For this review, take the finished solid that the model builds, in its own axes (mm). A direction names the side the tool comes from. Round coordinates to 2 decimals unless told otherwise and drop trailing zeros. Write each loop counter-clockwise with the first axis right and the second up, starting at its lowest first coordinate (ties: lowest second). Pieces come first, ordered by that corner, then holes.
from build123d import *

# Parameters (mm, degrees)
SKETCH1_R           = 40
SKETCH1_R_2         = 5
BOSS_EXTRUDE1_DEPTH = 5
SKETCH2_R           = 40
SKETCH2_R_2         = 38.5
SKETCH2_R_3         = 3
BOSS_EXTRUDE2_DEPTH = 15
SKETCH5_R           = 4
CUT_EXTRUDE1_DEPTH  = 5


with BuildPart() as part:
    # Sketch1 → Boss-Extrude1 (new body)
    with BuildSketch(Plane(origin=(0, 0, 0), x_dir=(1, 0, 0), z_dir=(0, 1, 0))):
        with Locations(Location((0, 0, 0), (0, 0, 270))):
            Circle(SKETCH1_R)
        with Locations(Location((-21, 21, 0), (0, 0, 270))):
            Circle(SKETCH1_R_2, mode=Mode.SUBTRACT)
        with Locations(Location((-21, -21, 0), (0, 0, 270))):
            Circle(SKETCH1_R_2, mode=Mode.SUBTRACT)
        with Locations(Location((21, -21, 0), (0, 0, 270))):
            Circle(SKETCH1_R_2, mode=Mode.SUBTRACT)
        with Locations(Location((21, 21, 0), (0, 0, 270))):
            Circle(SKETCH1_R_2, mode=Mode.SUBTRACT)
    extrude(amount=BOSS_EXTRUDE1_DEPTH)

    # Sketch2 → Boss-Extrude2 (add)
    # profile 1 of 7: a face of its own
    with BuildSketch(Plane(origin=(0, 5, 0), x_dir=(1, 0, 0), z_dir=(0, 1, 0))):
        with Locations(Location((0, 0, 0), (0, 0, 270))):
            Circle(SKETCH2_R)
        with Locations(Location((0, 0, 0), (0, 0, 270))):
            Circle(SKETCH2_R_2, mode=Mode.SUBTRACT)
    # profile 2 of 7: a face of its own
    with BuildSketch(Plane(origin=(0, 5, 0), x_dir=(1, 0, 0), z_dir=(0, 1, 0))):
        with Locations(Location((-12, -21, 0), (0, 0, 270))):
            Circle(SKETCH2_R_3)
    # profile 3 of 7: a face of its own
    with BuildSketch(Plane(origin=(0, 5, 0), x_dir=(1, 0, 0), z_dir=(0, 1, 0))):
        with Locations(Location((12, -21, 0), (0, 0, 270))):
            Circle(SKETCH2_R_3)
    # profile 4 of 7: a face of its own
    with BuildSketch(Plane(origin=(0, 5, 0), x_dir=(1, 0, 0), z_dir=(0, 1, 0))):
        with Locations(Location((21, -12, 0), (0, 0, 270))):
            Circle(SKETCH2_R_3)
    # profile 5 of 7: a face of its own
    with BuildSketch(Plane(origin=(0, 5, 0), x_dir=(1, 0, 0), z_dir=(0, 1, 0))):
        with Locations(Location((21, 12, 0), (0, 0, 270))):
            Circle(SKETCH2_R_3)
    # profile 6 of 7: a face of its own
    with BuildSketch(Plane(origin=(0, 5, 0), x_dir=(1, 0, 0), z_dir=(0, 1, 0))):
        with Locations(Location((12, 21, 0), (0, 0, 270))):
            Circle(SKETCH2_R_3)
    # profile 7 of 7: a face of its own
    with BuildSketch(Plane(origin=(0, 5, 0), x_dir=(1, 0, 0), z_dir=(0, 1, 0))):
        with Locations(Location((-12, 21, 0), (0, 0, 270))):
            Circle(SKETCH2_R_3)
    extrude(amount=BOSS_EXTRUDE2_DEPTH)

    # Sketch5 → Cut-Extrude1 (cut)
    with BuildSketch(Plane.XZ):
        with Locations(Location((-22, 0, 0), (0, 0, 270))):
            Circle(SKETCH5_R)
    extrude(amount=-CUT_EXTRUDE1_DEPTH, mode=Mode.SUBTRACT)


solid = part.part
(1) We need section A-A, the plane y = 15.5. Give the boundary of the cut face in (x, z).
Geometry check:
outline: circle Ø80 at (0, 0); circle Ø6 at (-12, -21); circle Ø6 at (-12, 21); circle Ø6 at (12, -21); circle Ø6 at (12, 21); circle Ø6 at (21, -12); circle Ø6 at (21, 12); hole circle Ø77 at (0, 0)
(2) Mouldability with a two-part tool opening along X and no side actions: class faces 1 (the face through (-12, 20, -21)), 2 (the face through (-39.05, 9.86, -8.67)), 3 (the face through (-37.584, 12.395, -8.346)) as pulls with the +X half, pulls with the -X half, needs draft (parallel to the pull), parting line crosses it, or undercut.
Geometry check:
face 1: needs draft
face 2: parting line crosses it
face 3: undercut
(3) For line 1 along X through (y, z) = (16.75, 1); line 2 along X through (y, z) = (1.4, 0); line 3 along X through (y, z) = (1.6, 21), list the stretches that pass through material, from the lowest coordinate up.
Geometry check:
line 1: x = -39.99 to -38.49, 38.49 to 39.99
line 2: x = -40 to -26, -18 to 40
line 3: x = -34.04 to -26, -16 to 16, 26 to 34.04
(4) We need section B-B, the plane z = 0. Give the boundary of the cut face in (x, y).
Geometry check:
outline: (-40, 0) - (-26, 0) - (-26, 5) - (-38.5, 5) - (-38.5, 20) - (-40, 20) - close; (-18, 0) - (40, 0) - (40, 20) - (38.5, 20) - (38.5, 5) - (-18, 5) - close
(5) We need section D-D, the plane z = 21. Give the boundary of the cut face in (x, y), and give its area (3 significant figures).
Geometry check:
outline: (-34.04, 0) - (-26, 0) - (-26, 5) - (-32.27, 5) - (-32.27, 20) - (-34.04, 20) - close; (-16, 0) - (16, 0) - (16, 5) - (15, 5) - (15, 20) - (9, 20) - (9, 5) - (-9, 5) - (-9, 20) - (-15, 20) - (-15, 5) - (-16, 5) - close; (26, 0) - (34.04, 0) - (34.04, 20) - (32.27, 20) - (32.27, 5) - (26, 5) - close
area: 474 mm2
(6) For pin 1 Ø10 at (x, y) = (-8, 11.5) entering from +Z; pin 2 Ø6 at (x, y) = (-7.5, 9.5) entering from +Z; pin 3 Ø1 at (x, z) = (-14.5, 13.5) entering from -Y; pin 4 Ø10.5 at (x, z) = (-22, 0) entering from +Y, all flat-tipped, find the tip position at first contact; note any pin that passes through.
Geometry check:
pin 1: stops at z = 39.89
pin 2: stops at z = 39.75
pin 3: stops at y = 0
pin 4: stops at y = 5
(7) We need section C-C, the plane x = -21. Give the boundary of the cut face in (y, z), and give its area (3 significant figures).
Geometry check:
outline: (0, -34.04) - (20, -34.04) - (20, -32.27) - (5, -32.27) - (5, -26) - (0, -26) - close; (0, -16) - (5, -16) - (5, -3.87) - (0, -3.87) - close; (0, 3.87) - (5, 3.87) - (5, 16) - (0, 16) - close; (0, 26) - (5, 26) - (5, 32.27) - (20, 32.27) - (20, 34.04) - (0, 34.04) - close
area: 255 mm2
(8) For faces 4 (the face through (21, 20, 12)), 5 (the face through (12, 12, 18)), list the 3-axis set-ups (+Z, -Z, +X, -X, +Y, -Y) from which the entire face can be reached by the end or side of a thin tool; tool diameter is ignored.
Geometry check:
face 4: +Z, -Z, +X, -X, +Y
face 5: +Y
